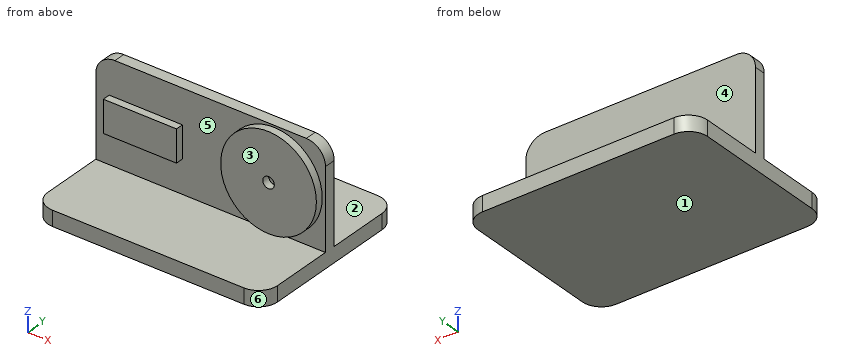
```python
from build123d import *

# Parameters (mm, degrees)
F1_DEPTH      = 4
F2_W          = 60
F2_H          = 30
F3_DEPTH      = 1.5
F3_DEPTH_BACK = 1.5
F4_R          = 5
F5_R          = 5
F6_R          = 12.5
F6_R_2        = 1.5
F6_W          = 19.108927
F6_H          = 8.373576
F7_DEPTH      = 2


with BuildPart() as f1:
    # F0 (on Top) → F1 (new body)
    with BuildSketch(Plane.XY):
        Polygon((-30, -22.77798), (30, -22.77798), (30, 0), (0, 0), (-30, 0), align=None)
        Polygon((0, 0), (30, 0), (30, 22.77798), (-30, 22.77798), (-30, 0), align=None)
    extrude(amount=F1_DEPTH)

    # F2 (on Front) → F3 (join, two sides)
    with BuildSketch(Plane.XZ) as f3_sk:
        with Locations((0, 15)):
            Rectangle(F2_W, F2_H)
    extrude(amount=F3_DEPTH)
    extrude(f3_sk.sketch, amount=-F3_DEPTH_BACK)

    # F4
    f4_edges = [f1.edges().sort_by_distance(p)[0] for p in [
        (-30, -22.77798, 2),
        (30, -22.77798, 2),
        (30, 22.77798, 2),
        (-30, 22.77798, 2),
    ]]
    fillet(f4_edges, radius=F4_R)

    # F5
    f5_edges = [f1.edges().sort_by_distance(p)[0] for p in [
        (-30, 0, 30),
        (30, 0, 30),
    ]]
    fillet(f5_edges, radius=F5_R)

    # F6 (on face) → F7 (join)
    with BuildSketch(Plane.XZ.offset(1.5)):
        with Locations((16.666592, 17)):
            Circle(F6_R)
        with Locations((16.666592, 17)):
            Circle(F6_R_2, mode=Mode.SUBTRACT)
        with Locations((-16.935061, 16.813212)):
            Rectangle(F6_W, F6_H)
    extrude(amount=F7_DEPTH)


solid = f1.part
```
Design review of the part built by this model. Coordinates are the model's own, in mm. Face numbers are marked on the shaded views. A direction names the side the tool comes from. Coordinates: 2 decimals unless noted, no trailing zeros. Loops run counter-clockwise (first coordinate to the right, second up) from the corner with the lowest first, then second, coordinate; pieces in that order, holes last. Notation, with made-up numbers: M 43,74 L 61,74 A25 cw 61,92 Z; hole C 0.25,43 d4. An arc over 180 degrees is marked long. One line per question, with ' | ' between items.
(1) We need section D-D (x = -20). Give the boundary of the cut face in (y, z), and give its area (3 significant figures).
Filled in:
outline: M -22.78,0 L 22.78,0 L 22.78,4 L 1.5,4 L 1.5,30 L -1.5,30 L -1.5,21 L -3.5,21 L -3.5,12.63 L -1.5,12.63 L -1.5,4 L -22.78,4 Z | area: 277 mm^2
(2) Machinability: for the marked faces 1, 2 and 3, which of the approach directions +Z, -Z, +X, -X, +Y, -Y give a long, thin tool a straight path to every point of the face, cutting with its end or side? Answer none if there is none.
Filled in:
face 1: -Z, +X, -X, +Y, -Y | face 2: +Z, +X, -X, +Y | face 3: +Z, +X, -X, -Y
(3) We need section B-B (z = 17). Give the boundary of the cut face in (x, y), and give its area (3 significant figures).
Filled in:
outline: M -30,-1.5 L -26.49,-1.5 L -26.49,-3.5 L -7.38,-3.5 L -7.38,-1.5 L 4.17,-1.5 L 4.17,-3.5 L 15.17,-3.5 L 15.17,-1.5 L 18.17,-1.5 L 18.17,-3.5 L 29.17,-3.5 L 29.17,-1.5 L 30,-1.5 L 30,1.5 L -30,1.5 Z | area: 262 mm^2
(4) Wall thickness on probe 1 along Z at (x, y) = (-16.5, -7); probe 2 along Y at (x, z) = (17.5, 22); probe 3 along Y at (x, z) = (8, 27.75): over which ranges is each line inside the solid? List them lowest first.
Filled in:
probe 1: z = 0 to 4 | probe 2: y = -3.5 to 1.5 | probe 3: y = -1.5 to 1.5
(5) We need section A-A (x = -3.5). Give the boundary of the cut face in (y, z), and give its area (3 significant figures).
Filled in:
outline: M -22.78,0 L 22.78,0 L 22.78,4 L 1.5,4 L 1.5,30 L -1.5,30 L -1.5,4 L -22.78,4 Z | area: 260 mm^2
(6) For pin 1 Ø10.5 at (x, y) = (3, 14) entering from +Z; pin 2 Ø7.5 at (x, z) = (10.5, 22.5) entering from -Y; pin 3 Ø1 at (y, z) = (-2.5, 26) entering from +X, all flat-tipped, find the tip position at first contact; note any pin that passes through.
Filled in:
pin 1: stops at z = 4 | pin 2: stops at y = -3.5 | pin 3: stops at x = 25.83
(7) We need section C-C (y = 12.5). Give the boundary of the cut face in (x, z), and give its area (3 significant figures).
Filled in:
outline: M -30,0 L 30,0 L 30,4 L -30,4 Z | area: 240 mm^2
(8) Draft analysis for pull direction X (two halves, no side actions). For the marked faces 4, 5 and 6, state which applies: released by +X, released by -X, zero draft, split by the parting line, or undercut.
Filled in:
face 4: zero draft | face 5: undercut | face 6: released by +X
